```python
from build123d import *

# Parameters (mm, degrees)
F1_DEPTH  = 51.562
F2_T      = -1.27
F4_D      = 5.2197
F4_DEPTH  = 0.762
F4_TIP    = 1.5681560866
F6_D      = 5.2197
F7_W      = 304.8
F7_H      = 304.8
F8_DEPTH  = 25.4
F10_D     = 5.2197
F10_DEPTH = 0.762
F10_TIP   = 1.5681560866


with BuildPart() as f1:
    # F0 (on Top) → F1 (new body)
    with BuildSketch(Plane.XY):
        Polygon((512.445, 360.045), (0, 360.045), (0, 0), (0, -360.045), (512.445, -360.045), align=None)
        Polygon((0, 0), (0, 360.045), (-512.445, 360.045), (-512.445, -360.045), (0, -360.045), align=None)
    extrude(amount=F1_DEPTH)

    # F2
    f2_openings = [f1.faces().sort_by_distance(p)[0] for p in [
        (0, 0, 51.562),
    ]]
    offset(amount=F2_T, openings=f2_openings)

    # F4
    with Locations(Plane.XZ.offset(360.045)):
        with Locations((-431.8, 7.112), (-215.9, 7.112), (0, 7.112), (215.9, 7.112), (431.8, 7.112)):
            Hole(F4_D / 2, depth=F4_DEPTH)
            with Locations((0, 0, -(F4_DEPTH + F4_TIP / 2))):  # 118° drill point
                Cone(0, F4_D / 2, F4_TIP, mode=Mode.SUBTRACT)

    # F6 (through all)
    with Locations(Plane(origin=(-512.445, 0, 0), x_dir=(0, -1, 0), z_dir=(-1, 0, 0))):
        with Locations((-304.8, 7.112), (-101.6, 7.112), (101.6, 7.112), (304.8, 7.112)):
            Hole(F6_D / 2)

    # F7 (on face) → F8 (cut)
    with BuildSketch(Plane(origin=(0, 0, 0), x_dir=(1, 0, 0), z_dir=(0, 0, -1))):
        with Locations((0, 133.35)):
            Rectangle(F7_W, F7_H)
    extrude(amount=-F8_DEPTH, mode=Mode.SUBTRACT)

    # F10
    with Locations(Plane(origin=(0, 360.045, 0), x_dir=(-1, 0, 0), z_dir=(0, 1, 0))):
        with Locations((-419.1, 14.2875), (-279.4, 14.2875), (-139.7, 14.2875), (0, 14.2875), (139.7, 14.2875), (279.4, 14.2875), (419.1, 14.2875)):
            Hole(F10_D / 2, depth=F10_DEPTH)
            with Locations((0, 0, -(F10_DEPTH + F10_TIP / 2))):  # 118° drill point
                Cone(0, F10_D / 2, F10_TIP, mode=Mode.SUBTRACT)


solid = f1.part
```
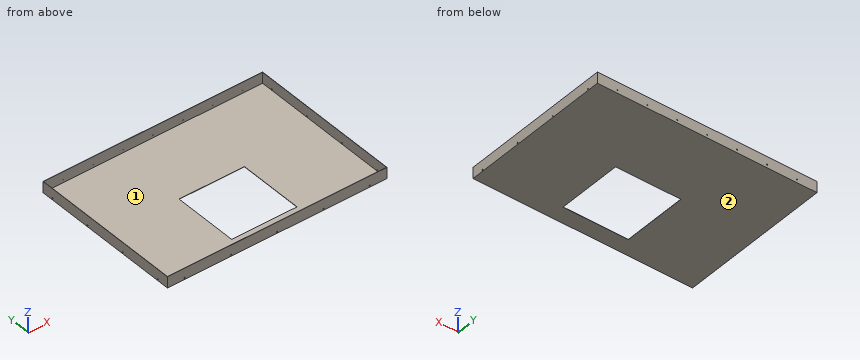
Input: part model. Units: mm. Frame: model coordinates. Face numbers are marked on the shaded views. Coordinates: 2 decimals unless noted, no trailing zeros. Loops run counter-clockwise (first coordinate to the right, second up) from the corner with the lowest first, then second, coordinate; pieces in that order, holes last. Notation, with made-up numbers: M -19.5,-22.5 L -2.5,-22.5 A22 cw -2.5,-0.5 Z; hole C 25,3.25 d3. An arc over 180 degrees is marked long. Answer in a Markdown table with one row per item.
1. Section D-D, the plane y = 49. Output: boundary loops of the cut face in (x, z) (3 decimals).
Response:
| item | result |
|---|---|
| outline | M -512.445,0 L 512.445,0 L 512.445,51.562 L 511.175,51.562 L 511.175,1.27 L -511.175,1.27 L -511.175,51.562 L -512.445,51.562 Z |
2. First-contact query: pin 1 (4.5 mm diameter, centred on y = 101.6, z = 7.112, fed in from +X). Flat tip, straight axial feed; report the tip coordinate or a pass-through.
Response:
| item | result |
|---|---|
| pin 1 | passes through |
3. Section C-C, the plane z = 39. Output: boundary loops of the cut face in (x, y) (3 decimals), then the cut area to 3 significant figures.
Response:
| item | result |
|---|---|
| outline | M -512.445,-360.045 L 512.445,-360.045 L 512.445,360.045 L -512.445,360.045 Z; hole M -511.175,-358.775 L 511.175,-358.775 L 511.175,358.775 L -511.175,358.775 Z |
| area | 4,430 mm2 |
4. Draft query along X for the marked faces 1 and 2. Return one class per face: pulls with the +X half, pulls with the -X half, needs draft (parallel to the pull), parting line crosses it, or undercut.
Response:
| item | result |
|---|---|
| face 1 | undercut |
| face 2 | needs draft |
5. Section A-A, the plane y = -147.5. Output: boundary loops of the cut face in (x, z) (3 decimals).
Response:
| item | result |
|---|---|
| outline | M -512.445,0 L -152.4,0 L -152.4,1.27 L -511.175,1.27 L -511.175,51.562 L -512.445,51.562 Z; M 152.4,0 L 512.445,0 L 512.445,51.562 L 511.175,51.562 L 511.175,1.27 L 152.4,1.27 Z |
6. Section B-B, the plane x = 120. Output: boundary loops of the cut face in (y, z) (3 decimals).
Response:
| item | result |
|---|---|
| outline | M -360.045,0 L -285.75,0 L -285.75,1.27 L -358.775,1.27 L -358.775,51.562 L -360.045,51.562 Z; M 19.05,0 L 360.045,0 L 360.045,51.562 L 358.775,51.562 L 358.775,1.27 L 19.05,1.27 Z |
7. Material intervals for line 1 (X direction, y = 248, z = 45) (3 decimals); line 2 (Y direction, x = 18, z = 45.5) (3 decimals); line 3 (Z direction, x = -511.95, y = -101.6), sorted ascending.
Response:
| item | result |
|---|---|
| line 1 | x = -512.445 to -511.175, 511.175 to 512.445 |
| line 2 | y = -360.045 to -358.775, 358.775 to 360.045 |
| line 3 | z = 0 to 4.5, 9.72 to 51.56 |
